```python
from build123d import *

# Parameters (mm, degrees)
F0_R     = 6.35
F0_R_2   = 4.7625
F1_DEPTH = 25.4
F2_R     = 2.54
F3_DEPTH = 152.4
F4_R     = 4.7625
F5_DEPTH = 25.4


with BuildPart() as f1:
    # F0 (on Front) → F1 (new body)
    with BuildSketch(Plane.XZ):
        Circle(F0_R)
        Circle(F0_R_2, mode=Mode.SUBTRACT)
    extrude(amount=F1_DEPTH)

    # F2 (on Top) → F3 (join)
    with BuildSketch(Plane.XY):
        with Locations((0, -12.7)):
            Circle(F2_R)
    extrude(amount=-F3_DEPTH)

    # F4 (on face) → F5 (cut)
    with BuildSketch(Plane.XZ.offset(25.4)):
        Circle(F4_R)
    extrude(amount=-F5_DEPTH, mode=Mode.SUBTRACT)


solid = f1.part
```
Geometry check sheet. Reference: the model listing, model coordinates, mm. A direction names the side the tool comes from. Give positions to 0.01 mm unless a question says otherwise; leave off trailing zeros. Loops run counter-clockwise (first coordinate to the right, second up) from the corner with the lowest first, then second, coordinate; pieces in that order, holes last. Notation, with made-up numbers: M 33,-32 L 90,-32 A31 cw 90,6 Z; hole C 54.5,-33.75 d6. An arc over 180 degrees is marked long. Write item = value, one per line. Start each with the question number.
1. Section check B-B, the plane x = 0. Enter the section's corners in (y, z).
2. Section check D-D, the plane z = -100.5. Enter the section's corners in (x, y).
3. Tool access check on faces 1 (the face through (0, -13, -152.4)), 2 (the face through (-0.55, -15.18, -78.08)). Record the directions out of +Z, -Z, +X, -X, +Y, -Y that give a thin tool (end or side, any length) a straight path to the whole face; none if there is none.
4. Go/stop test with flat-tipped pins: P1, Ø8, axis at y = -17, z = -19.5, coming from the -X side; P2, Ø1.5, axis at x = -1.5, y = -15.5, coming from the +Z side; P3, Ø6, axis at x = 1, z = -62, coming from the +Y side. Record where each tip stops, or that it passes through.
5. Section check A-A, the plane z = 0. Enter the section's corners in (x, y), plus the area to 3 significant figures.
6. Thickness scan on probe 1 along Z at (x, y) = (0, -6.5); probe 2 along Z at (x, y) = (1.75, -21.75); probe 3 along Y at (x, z) = (-2.25, -49.5). Record the ranges inside material, lowest first.
Values follow:
q1.outline = M -25.4,-6.35 L -15.24,-6.35 L -15.24,-152.4 L -10.16,-152.4 L -10.16,-6.35 L 0,-6.35 L 0,-4.76 L -25.4,-4.76 Z; M -25.4,4.76 L 0,4.76 L 0,6.35 L -25.4,6.35 Z
q2.outline = C 0,-12.7 d5.08
q3.face_1 = -Z, +X, -X, +Y, -Y
q3.face_2 = -Z
q4.P1 = -2.52
q4.P2 = 6.31
q4.P3 = -10.16
q5.outline = M -6.35,-25.4 L -4.76,-25.4 L -4.76,0 L -6.35,0 Z; M 4.76,-25.4 L 6.35,-25.4 L 6.35,0 L 4.76,0 Z
q5.area = 80.6 mm^2
q6.probe_1 = -6.35 to -4.76, 4.76 to 6.35
q6.probe_2 = -6.1 to -4.43, 4.43 to 6.1
q6.probe_3 = -13.88 to -11.52
